Autodesk Inventor part; units mm, degrees
ref_plane "Plan de construction1" through (14.5, 0, 0) normal (1, 0, 0) x (0, 1, 0)
ref_plane "YZ Plane" through (0, 0, 0) normal (1, 0, 0) x (0, 1, 0)
ref_plane "XZ Plane" through (0, 0, 0) normal (0, 1, 0) x (-1, 0, 0)
sketch "Esquisse1" plane through (0, 0, 0) normal (1, 0, 0) x (0, 1, 0)
  line L0 (11.9, 7.9) -> (-11.9, 7.9)
  line L1 (-11.9, 7.9) -> (-11.9, -7.9)
  line L2 (-11.9, -7.9) -> (11.9, -7.9)
  line L3 (11.9, -7.9) -> (11.9, 7.9)
  point P0 (0, 0)
  point P1 (11.9, 0)
  point P2 (0, -7.9)
  dimension "d0" = 23.8
  dimension "d3" = 15.8
extrude "Extrusion1" add sketch "Esquisse1" along normal mid plane 3.2
sketch "Esquisse2" plane through (1.6, 0, 0) normal (1, 0, 0) x (0, 0, -1)
  circle A0 centre (0, 0) radius 8.7
  line L0 (7.9, -11.9) -> (7.9, 11.9)
  line L1 (7.9, 3.6442) -> (0, 0)
  line L2 (0, 0) -> (7.9, -3.6442)
  line L3 (0, 0) -> (-7.9, -3.6442)
  line L4 (-7.9, 11.9) -> (-7.9, -11.9)
  line L5 (0, 0) -> (-7.9, 3.6442)
  line L6 (0, 0) -> (3.6423, -7.9008)
  line L7 (0, 0) -> (-3.6423, -7.9008)
  line L8 (0, 0) -> (3.6423, 7.9008)
  line L9 (0, 0) -> (-3.6423, 7.9008)
  line L10 (3.6423, 7.9008) -> (-3.6423, 7.9008) construction
  line L11 (3.6423, -7.9008) -> (-3.6423, -7.9008) construction
  line L12 (0, -7.9008) -> (0, 7.9008) construction
  circle A1 centre (0, 0) radius 5.5
  point P0 (2.3026, 4.9948)
  point P1 (4.9943, 2.3038)
  point P2 (-4.9943, 2.3038)
  point P3 (-2.3026, 4.9948)
  point P4 (-2.3026, -4.9948)
  point P5 (-4.9943, -2.3038)
  point P6 (4.9943, -2.3038)
  point P7 (2.3026, -4.9948)
  dimension "d4" = 17.4
  dimension "d7" = 49.5
  dimension "d8" = 49.5
  dimension "d9" = 11
extrude "Extrusion3" add sketch "Esquisse2" along normal blind 11 contours L1 A1 L8 A0 | A0 L6 A1 L2 | L9 A1 L5 A0 | A0 L3 A1 L7
sketch "Esquisse3" plane through (1.6, 0, 0) normal (1, 0, 0) x (0, 0, -1)
  line L0 (0, -7.9) -> (0, -17.3183) construction
  line L1 (-2, -7.9) -> (-2, -17.3183)
  line L2 (2, -17.3183) -> (2, -7.9)
  arc A0 (2, -7.9) -> (-2, -7.9) centre (0, -7.9) ccw
  arc A1 (-2, -17.3183) -> (2, -17.3183) centre (0, -17.3183) ccw
  line L3 (-7.9, -11.9) -> (7.9, -11.9)
  line L4 (0, -25.5619) -> (0, 18.1437)
  point P0 (0, 0)
  point P1 (0, -12.6091)
  point P2 (2, -11.9)
  point P3 (-2, -11.9)
  dimension "d12" = 4
  dimension "d13" = 4
extrude "Extrusion4" cut sketch "Esquisse3" against normal blind 11 contours A0 L4 L3 L1 | A0 L2 L3 L4
mirror "Symétrie1" about plane through (0, 0, 0) normal (0, 1, 0) of "Extrusion4"
sketch "Esquisse4" plane through (0, 0, 0) normal (0, 0, 1) x (1, 0, 0)
  circle A0 centre (8.5, 0) radius 6
  line L0 (14.5, 0) -> (-1.6, 0)
  line L1 (-1.6, -11.9) -> (-1.6, 11.9)
  point P0 (0, 0)
  point P1 (2.5, 0)
  dimension "d16" = 12
  dimension "d17" = 16.1
revolve "Révolution1" add sketch "Esquisse4" angle 360 about axis through (14.5, 0, 0) along (-1, 0, 0) picked at (6.7291, -0.9294) contours A0 L0
fillet "Congé1" radius 2 4 edges at (0, 11.9, 7.9) (0, 11.9, -7.9) (0, -11.9, -7.9) (0, -11.9, 7.9)
ref_plane "Plan de construction1" through (14.5, 0, 0) normal (1, 0, 0) x (0, 1, 0)
properties part number "Roue_libre"
Read the model definition and answer for the solid it produces. Units are mm, in the model's axes. A direction names the side the tool comes from. Coordinates: 2 decimals unless noted, no trailing zeros. Loops run counter-clockwise (first coordinate to the right, second up) from the corner with the lowest first, then second, coordinate; pieces in that order, holes last. Notation, with made-up numbers: (44, -14) - (52, -14) arc R18 ccw to (52, 3) - close; hole circle Ø7 at (-1, 75). An arc over 180 degrees is marked (long way). Answer in a Markdown table with one row per item.
Q1. Given P1, Ø2, axis at x = 11, y = -6.5, coming from the +Z side; P2, Ø1.6, axis at x = 0.5, y = 10.5, coming from the +Z side; P3, Ø2, axis at x = 6.5, z = 5.5, coming from the +Y side; P4, Ø3, axis at x = 5.5, y = 8, coming from the +Z side, each flat-ended and moving along its own axis, determine where each tip first touches the part or whether it passes through.
Here are the results:
| item | result |
|---|---|
| P1 | stops at z = 6.74 |
| P2 | stops at z = 7.9 |
| P3 | stops at y = 7.45 |
| P4 | stops at z = 5.78 |
Q2. Straight lines are drawn through the part: line 1 along Y through (x, z) = (4.5, -3.25); line 2 along X through (y, z) = (6.5, -5); line 3 along X through (y, z) = (9, -2.25). For each, find the intervals that lie inside material, in ascending order. Write a range as [from, to].
Here are the results:
| item | result |
|---|---|
| line 1 | y = [-7.05, -4.44], [-3.07, 3.07], [4.44, 7.05] |
| line 2 | x = [-1.6, 12.6] |
| line 3 | x = [-1.6, 1.6] |
Q3. Find section D-D on x = 9.5. Write down the section's boundary in (y, z), plus the area to 3 significant figures.
Here are the results:
| item | result |
|---|---|
| outline | (-7.9, -3.64) arc R8.7 ccw to (-3.64, -7.9) - (-2.48, -5.37) arc R5.92 ccw to (2.48, -5.37) - (3.64, -7.9) arc R8.7 ccw to (7.9, -3.64) - (5.37, -2.48) arc R5.92 ccw to (5.37, 2.48) - (7.9, 3.64) arc R8.7 ccw to (3.64, 7.9) - (2.48, 5.37) arc R5.92 ccw to (-2.48, 5.37) - (-3.64, 7.9) arc R8.7 ccw to (-7.9, 3.64) - (-5.37, 2.48) arc R5.92 ccw to (-5.37, -2.48) - close |
| area | 167 mm^2 |
Q4. The mould has two halves that part along Y. Classify faces 1 (the cylindrical face through (11.74, -3.91, 3.87)), 2 (the flat face through (0, 10, -2)), 3 (the flat face through (0, 11.9, 4)): pulls with the +Y half, pulls with the -Y half, needs draft (parallel to the pull), parting line crosses it, or undercut.
Here are the results:
| item | result |
|---|---|
| face 1 | undercut |
| face 2 | needs draft |
| face 3 | pulls with the +Y half |
Q5. Find section C-C on z = -0.75. Write down the section's boundary in (x, y).
Here are the results:
| item | result |
|---|---|
| outline | (-1.6, -6.05) - (1.6, -6.05) - (1.6, 6.05) - (-1.6, 6.05) - close; circle Ø11.91 at (8.5, 0) |
Q6. Find section B-B on x = 12.25. Write down the section's boundary in (y, z).
Here are the results:
| item | result |
|---|---|
| outline | (-7.9, -3.64) arc R8.7 ccw to (-3.64, -7.9) - (-2.3, -4.99) arc R5.5 cw to (-4.99, -2.3) - close; (-7.9, 3.64) - (-4.99, 2.3) arc R5.5 cw to (-2.3, 4.99) - (-3.64, 7.9) arc R8.7 ccw to start; circle Ø9.37 at (0, 0); (2.3, -4.99) - (3.64, -7.9) arc R8.7 ccw to (7.9, -3.64) - (4.99, -2.3) arc R5.5 cw to start; (2.3, 4.99) arc R5.5 cw to (4.99, 2.3) - (7.9, 3.64) arc R8.7 ccw to (3.64, 7.9) - close |
Q7. Find section A-A on y = -5.5. Write down the section's boundary in (x, z).
Here are the results:
| item | result |
|---|---|
| outline | (-1.6, -7.9) - (1.6, -7.9) - (1.6, -6.74) - (12.6, -6.74) - (12.6, -2.54) - (1.6, -2.54) - (1.6, 2.54) - (12.6, 2.54) - (12.6, 6.74) - (1.6, 6.74) - (1.6, 7.9) - (-1.6, 7.9) - close; circle Ø4.8 at (8.5, 0) |
Q8. For faces 4 (the cylindrical face through (7.023, 6.122, 6.181)), 5 (the flat face through (0, -10, 2)), 6 (the cylindrical face through (7.023, -6.122, -6.181)), determine the directions among +Z, -Z, +X, -X, +Y, -Y from which every point of the face is accessible in a straight line to the end or side of a thin tool.
Here are the results:
| item | result |
|---|---|
| face 4 | +Z, +X, +Y |
| face 5 | +X, -X, -Y |
| face 6 | -Z, +X, -Y |
